Here's how the part is built. I have some questions about the finished solid (model axes, mm). A direction names the side the tool comes from. Coordinates: 2 decimals unless noted, no trailing zeros. Loops run counter-clockwise (first coordinate to the right, second up) from the corner with the lowest first, then second, coordinate; pieces in that order, holes last. Notation, with made-up numbers: (26, -19) -> (54, -19) arc R15 ccw to (54, 7) -> close; hole circle Ø8 at (69.25, -6). An arc over 180 degrees is marked (long way). Answer as a JSON object with one key per item and string values. Group by question number.
Q1. I need wall thicknesses on line 1 (X direction, y = 14, z = -51); line 2 (Y direction, x = 8.5, z = -65.5); line 3 (Y direction, x = 21.5, z = -54). Which ranges of each line are inside material? Lowest first, please.
Q2. I'm going to push flat-ended pins straight in: pin 1 (1.9 mm diameter, centred on x = 10, z = -65.5, fed in from +Y); pin 2 (2.5 mm diameter, centred on y = 12.5, z = -49.5, fed in from -X); pin 3 (4 mm diameter, centred on x = 11, z = -42, fed in from +Y). Where does each tip first touch, or does it pass through?
Q3. On a 3-axis mill with a long thin cutter (end or side, diameter ignored), from which of +Z, -Z, +X, -X, +Y, -Y can I reach the whole of each face in a straight line? I mean faces 1 (the flat face through (13, 10, -5)), 2 (the cylindrical face through (25.9, 13.18, -0.86)), 3 (the flat face through (25, 13, -35)), 4 (the cylindrical face through (14.06, 9.1, -69.14)). Say none if no direction works.
Q4. I want a section at B-B on y = 12.5. Write out the boundary of the cut face in (x, z), then the cut area to 3 significant figures.
Q5. Thinking about a two-plate mould opening in Z: for faces 5 (the cylindrical face through (49.1, 8.38, -0.86)), 6 (the flat face through (50, 8, -35)), 7 (the flat face through (30, 6, -70)), 8 (the cylindrical face through (14, 8, -35)), which applies, released by +Z, released by -Z, zero draft, split by the parting line, or undercut?
Q6. I want a section at A-A on x = 15. Write out the boundary of the cut face in (y, z).
```python
from build123d import *

# Parameters (mm, degrees)
SKETCH1_W           = 50
SKETCH1_H           = 70
BOSS_EXTRUDE1_DEPTH = 20
CUT_EXTRUDE1_DEPTH  = 25
FILLET1_R           = 3


with BuildPart() as part:
    # Sketch1 → Boss-Extrude1 (new body)
    with BuildSketch(Plane(origin=(0, 0, 0), x_dir=(1, 0, 0), z_dir=(0, 1, 0))):
        with Locations((25, 35)):
            Rectangle(SKETCH1_W, SKETCH1_H)
    extrude(amount=BOSS_EXTRUDE1_DEPTH)

    # Sketch3 → Cut-Extrude1 (cut)
    with BuildSketch(Plane.ZY):
        with BuildLine():
            Line((-70, 20), (0, 20))
            Line((0, 20), (0, 10))
            Line((0, 10), (-6.786528041, 10))
            ThreePointArc((-6.786528041, 10), (-35, 8), (-63.213471959, 10))
            Line((-63.213471959, 10), (-70, 10))
            Line((-70, 10), (-70, 20))
        make_face()
    extrude(amount=-CUT_EXTRUDE1_DEPTH, mode=Mode.SUBTRACT)

    # Fillet1
    # the kernel refuses this fillet: 3 mm, written as the material it takes off along each edge
    with BuildSketch(Plane(origin=(28, 17, -67), x_dir=(-1, 0, 0), z_dir=(0, 1, 0))) as fillet1_piece_1_section:
        Polygon((0, 0), (FILLET1_R, 0), (FILLET1_R, -FILLET1_R), (0, -FILLET1_R), align=None)
    fillet1_piece_1 = extrude(amount=FILLET1_R, mode=Mode.PRIVATE)
    fillet1_piece_1 = fillet1_piece_1 - Plane(origin=(28, 17, -67), x_dir=(0.7071067811865475, 0, 0.7071067811865475), z_dir=(0, 1, 0)) * Sphere(FILLET1_R, mode=Mode.PRIVATE)
    add(fillet1_piece_1, mode=Mode.SUBTRACT)
    with BuildSketch(Plane(origin=(28, 17, -3), x_dir=(0, 1, 0), z_dir=(0, 0, 1))) as fillet1_piece_2_section:
        Polygon((0, 0), (FILLET1_R, 0), (FILLET1_R, FILLET1_R), (0, FILLET1_R), align=None)
    fillet1_piece_2 = extrude(amount=FILLET1_R, mode=Mode.PRIVATE)
    fillet1_piece_2 = fillet1_piece_2 - Plane(origin=(28, 17, -3), x_dir=(0.7071067811865475, -0.7071067811865475, 0), z_dir=(0, 0, 1)) * Sphere(FILLET1_R, mode=Mode.PRIVATE)
    add(fillet1_piece_2, mode=Mode.SUBTRACT)
    with BuildSketch(Plane(origin=(47, 17, -67), x_dir=(0, 1, 0), z_dir=(1, 0, 0))) as fillet1_piece_3_section:
        Polygon((0, 0), (FILLET1_R, 0), (FILLET1_R, -FILLET1_R), (0, -FILLET1_R), align=None)
    fillet1_piece_3 = extrude(amount=FILLET1_R, mode=Mode.PRIVATE)
    fillet1_piece_3 = fillet1_piece_3 - Plane(origin=(47, 17, -67), x_dir=(0, -0.7071067811865475, 0.7071067811865475), z_dir=(1, 0, 0)) * Sphere(FILLET1_R, mode=Mode.PRIVATE)
    add(fillet1_piece_3, mode=Mode.SUBTRACT)
    with BuildSketch(Plane(origin=(47, 17, -3), x_dir=(1, 0, 0), z_dir=(0, 0, 1))) as fillet1_piece_4_section:
        Polygon((0, 0), (FILLET1_R, 0), (FILLET1_R, FILLET1_R), (0, FILLET1_R), align=None)
    fillet1_piece_4 = extrude(amount=FILLET1_R, mode=Mode.PRIVATE)
    fillet1_piece_4 = fillet1_piece_4 - Plane(origin=(47, 17, -3), x_dir=(-0.7071067811865475, -0.7071067811865475, 0), z_dir=(0, 0, 1)) * Sphere(FILLET1_R, mode=Mode.PRIVATE)
    add(fillet1_piece_4, mode=Mode.SUBTRACT)
    with BuildSketch(Plane(origin=(25, 10, -70), x_dir=(0, 0, 1), z_dir=(0, 1, 0))) as fillet1_piece_5:
        with BuildLine():
            CenterArc((FILLET1_R, FILLET1_R), FILLET1_R, 180, 90)
            Line((0, FILLET1_R), (0, 0))
            Line((0, 0), (FILLET1_R, 0))
        make_face()
    extrude(amount=7, mode=Mode.SUBTRACT)
    with BuildSketch(Plane(origin=(25, 17, 0), x_dir=(1, 0, 0), z_dir=(0, -1, 0))) as fillet1_piece_6:
        with BuildLine():
            CenterArc((FILLET1_R, -FILLET1_R), FILLET1_R, 90, 90)
            Line((0, -FILLET1_R), (0, 0))
            Line((0, 0), (FILLET1_R, 0))
        make_face()
    extrude(amount=7, mode=Mode.SUBTRACT)
    with BuildSketch(Plane(origin=(-7.5, 10, -70), x_dir=(0, -1, 0), z_dir=(1, 0, 0))) as fillet1_piece_7:
        with BuildLine():
            CenterArc((FILLET1_R, -FILLET1_R), FILLET1_R, 90, 90)
            Line((0, -FILLET1_R), (0, 0))
            Line((0, 0), (FILLET1_R, 0))
        make_face()
    extrude(amount=32.5, mode=Mode.SUBTRACT)
    with BuildSketch(Plane(origin=(0, 208, -35), x_dir=(0, -0.9840151144884159, 0.17808496415573608), z_dir=(0, 0.17808496415573608, 0.9840151144884159))) as fillet1_piece_8:
        with BuildLine():
            CenterArc((200 + FILLET1_R, FILLET1_R), FILLET1_R, 180, 90)
            Line((200, FILLET1_R), (200, 0))
            Line((200, 0), (200 + FILLET1_R, 0))
        make_face()
    revolve(axis=Axis((0, 208, -35), (1, 0, 0)), revolution_arc=20.516468422, mode=Mode.SUBTRACT)
    with BuildSketch(Plane(origin=(-7.5, 10, 0), x_dir=(0, -1, 0), z_dir=(1, 0, 0))) as fillet1_piece_9:
        with BuildLine():
            CenterArc((FILLET1_R, FILLET1_R), FILLET1_R, 180, 90)
            Line((0, FILLET1_R), (0, 0))
            Line((0, 0), (FILLET1_R, 0))
        make_face()
    extrude(amount=32.5, mode=Mode.SUBTRACT)
    with BuildSketch(Plane(origin=(47, 20, -70), x_dir=(0, 0, 1), z_dir=(-1, 0, 0))) as fillet1_piece_10:
        with BuildLine():
            CenterArc((FILLET1_R, -FILLET1_R), FILLET1_R, 90, 90)
            Line((0, -FILLET1_R), (0, 0))
            Line((0, 0), (FILLET1_R, 0))
        make_face()
    extrude(amount=19, mode=Mode.SUBTRACT)
    with BuildSketch(Plane(origin=(50, 20, -3), x_dir=(0, -1, 0), z_dir=(0, 0, -1))) as fillet1_piece_11:
        with BuildLine():
            CenterArc((FILLET1_R, FILLET1_R), FILLET1_R, 180, 90)
            Line((0, FILLET1_R), (0, 0))
            Line((0, 0), (FILLET1_R, 0))
        make_face()
    extrude(amount=64, mode=Mode.SUBTRACT)
    with BuildSketch(Plane(origin=(28, 20, 0), x_dir=(0, -1, 0), z_dir=(1, 0, 0))) as fillet1_piece_12:
        with BuildLine():
            CenterArc((FILLET1_R, FILLET1_R), FILLET1_R, 180, 90)
            Line((0, FILLET1_R), (0, 0))
            Line((0, 0), (FILLET1_R, 0))
        make_face()
    extrude(amount=19, mode=Mode.SUBTRACT)
    with BuildSketch(Plane(origin=(25, 20, -67), x_dir=(1, 0, 0), z_dir=(0, 0, 1))) as fillet1_piece_13:
        with BuildLine():
            CenterArc((FILLET1_R, -FILLET1_R), FILLET1_R, 90, 90)
            Line((0, -FILLET1_R), (0, 0))
            Line((0, 0), (FILLET1_R, 0))
        make_face()
    extrude(amount=64, mode=Mode.SUBTRACT)
    with BuildSketch(Plane(origin=(0, -7.5, 0), x_dir=(1, 0, 0), z_dir=(0, 1, 0)), Plane(origin=(0, -7.5, -70), x_dir=(0, 0, 1), z_dir=(0, 1, 0))) as fillet1_piece_14:
        with BuildLine():
            CenterArc((FILLET1_R, FILLET1_R), FILLET1_R, 180, 90)
            Line((0, FILLET1_R), (0, 0))
            Line((0, 0), (FILLET1_R, 0))
        make_face()
    extrude(amount=25, mode=Mode.SUBTRACT)
    with BuildSketch(Plane(origin=(50, -7.5, -70), x_dir=(0, 0, 1), z_dir=(0, 1, 0)), Plane(origin=(50, -7.5, 0), x_dir=(-1, 0, 0), z_dir=(0, 1, 0))) as fillet1_piece_15:
        with BuildLine():
            CenterArc((FILLET1_R, -FILLET1_R), FILLET1_R, 90, 90)
            Line((0, -FILLET1_R), (0, 0))
            Line((0, 0), (FILLET1_R, 0))
        make_face()
    extrude(amount=24.5, mode=Mode.SUBTRACT)
    with BuildSketch(Plane(origin=(25, 2.5, -70), x_dir=(0, 0, 1), z_dir=(0, 1, 0))) as fillet1_piece_16a_section:
        with BuildLine():
            CenterArc((FILLET1_R, FILLET1_R), FILLET1_R, 180, 90)
            Line((0, FILLET1_R), (0, 0))
            Line((0, 0), (FILLET1_R, 0))
        make_face()
    fillet1_piece_16a = extrude(amount=14.5, mode=Mode.PRIVATE)
    fillet1_piece_16a = split(fillet1_piece_16a, bisect_by=Plane(origin=(25.679185343, 10, -69.320814657), z_dir=(0, -1, 0)), keep=Keep.TOP, mode=Mode.PRIVATE)
    with BuildSketch(Plane(origin=(-7.5, 10, -70), x_dir=(0, -1, 0), z_dir=(1, 0, 0))) as fillet1_piece_16b_section:
        with BuildLine():
            CenterArc((FILLET1_R, -FILLET1_R), FILLET1_R, 90, 90)
            Line((0, -FILLET1_R), (0, 0))
            Line((0, 0), (FILLET1_R, 0))
        make_face()
    fillet1_piece_16b = extrude(amount=40, mode=Mode.PRIVATE)
    fillet1_piece_16b = split(fillet1_piece_16b, bisect_by=Plane(origin=(25, 9.320814657, -69.320814657), z_dir=(1, 0, 0)), keep=Keep.TOP, mode=Mode.PRIVATE)
    fillet1_piece_16 = fillet1_piece_16a & fillet1_piece_16b
    add(fillet1_piece_16, mode=Mode.SUBTRACT)
    with BuildSketch(Plane(origin=(25, 17, 0), x_dir=(1, 0, 0), z_dir=(0, -1, 0))) as fillet1_piece_17a_section:
        with BuildLine():
            CenterArc((FILLET1_R, -FILLET1_R), FILLET1_R, 90, 90)
            Line((0, -FILLET1_R), (0, 0))
            Line((0, 0), (FILLET1_R, 0))
        make_face()
    fillet1_piece_17a = extrude(amount=14.5, mode=Mode.PRIVATE)
    fillet1_piece_17a = split(fillet1_piece_17a, bisect_by=Plane(origin=(25.679185343, 10, -0.679185343), z_dir=(0, -1, 0)), keep=Keep.TOP, mode=Mode.PRIVATE)
    with BuildSketch(Plane(origin=(-7.5, 10, 0), x_dir=(0, -1, 0), z_dir=(1, 0, 0))) as fillet1_piece_17b_section:
        with BuildLine():
            CenterArc((FILLET1_R, FILLET1_R), FILLET1_R, 180, 90)
            Line((0, FILLET1_R), (0, 0))
            Line((0, 0), (FILLET1_R, 0))
        make_face()
    fillet1_piece_17b = extrude(amount=40, mode=Mode.PRIVATE)
    fillet1_piece_17b = split(fillet1_piece_17b, bisect_by=Plane(origin=(25, 9.320814657, -0.679185343), z_dir=(1, 0, 0)), keep=Keep.TOP, mode=Mode.PRIVATE)
    fillet1_piece_17 = fillet1_piece_17a & fillet1_piece_17b
    add(fillet1_piece_17, mode=Mode.SUBTRACT)


solid = part.part
```
Result set:
{
 "1": {"line 1": "x = 25 to 50", "line 2": "y = 0 to 10", "line 3": "y = 0 to 8.9"},
 "2": {"pin 1": "stops at y = 10", "pin 2": "stops at x = 25", "pin 3": "stops at y = 8.2"},
 "3": {"face 1": "+Z, -Z, -X, +Y", "face 2": "+Z, -X, +Y", "face 3": "-X, +Y", "face 4": "-Z, -X, +Y"},
 "4": {"outline": "(25, -67) arc R3 ccw to (28, -70) -> (47, -70) arc R3 ccw to (50, -67) -> (50, -3) arc R3 ccw to (47, 0) -> (28, 0) arc R3 ccw to (25, -3) -> close", "area": "1,740 mm²"},
 "5": {"face 5": "released by +Z", "face 6": "zero draft", "face 7": "released by -Z", "face 8": "undercut"},
 "6": {"outline": "(0, -70) -> (7, -70) arc R3 ccw to (10, -67) -> (10, -63.21) arc R200 cw to (10, -6.79) -> (10, -3) arc R3 ccw to (7, 0) -> (0, 0) -> close"}
}
